Verification items for the finished model (mm, model axes). Face numbers are marked on the shaded views. A direction names the side the tool comes from. Give positions to 0.01 mm unless a question says otherwise; leave off trailing zeros. Loops run counter-clockwise (first coordinate to the right, second up) from the corner with the lowest first, then second, coordinate; pieces in that order, holes last. Notation, with made-up numbers: (-9, -20.75) -> (47, -20.75) arc R11 ccw to (47, -11.75) -> close; hole circle Ø5 at (50.25, 64). An arc over 180 degrees is marked (long way). Use one line per item in the form item = value. Start each with the question number.
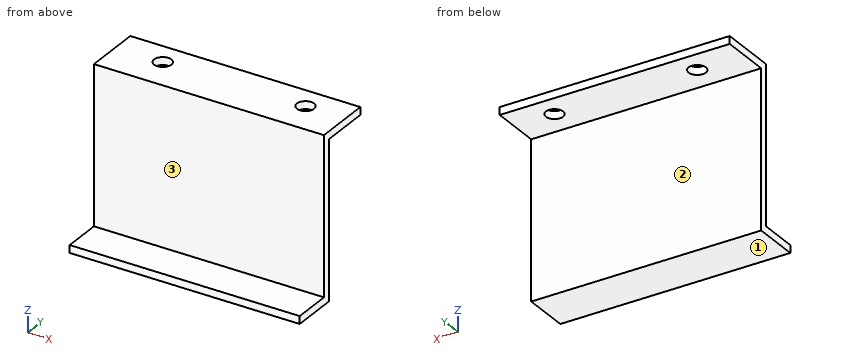
from build123d import *

# Parameters (mm, degrees)
SKETCH1_W            = 60
SKETCH1_H            = 20
BOSS_EXTRUDE1_DEPTH  = 43
SKETCH2_W            = 60
SKETCH2_H            = 8
CUT_EXTRUDE1_DEPTH   = 41
SKETCH3_W            = 60
SKETCH3_H            = 10
CUT_EXTRUDE2_DEPTH   = 41
SKETCH4_W            = 60
SKETCH4_H            = 2
BOSS_EXTRUDE2_DEPTH  = 5
M4_CLEARANCE_HOLE1_D = 4.5


with BuildPart() as part:
    # Sketch1 → Boss-Extrude1 (new body)
    with BuildSketch(Plane.XY):
        Rectangle(SKETCH1_W, SKETCH1_H)
    extrude(amount=BOSS_EXTRUDE1_DEPTH)

    # Sketch2 → Cut-Extrude1 (cut)
    with BuildSketch(Plane(origin=(0, 0, 0), x_dir=(-1, 0, 0), z_dir=(0, 0, -1))):
        with Locations((0, 6)):
            Rectangle(SKETCH2_W, SKETCH2_H)
    extrude(amount=-CUT_EXTRUDE1_DEPTH, mode=Mode.SUBTRACT)

    # Sketch3 → Cut-Extrude2 (cut)
    with BuildSketch(Plane.XY.offset(43)):
        with Locations((0, -5)):
            Rectangle(SKETCH3_W, SKETCH3_H)
    extrude(amount=-CUT_EXTRUDE2_DEPTH, mode=Mode.SUBTRACT)

    # Sketch4 → Boss-Extrude2 (add)
    with BuildSketch(Plane(origin=(0, 10, 0), x_dir=(1, 0, 0), z_dir=(0, 1, 0))):
        with Locations((0, -42)):
            Rectangle(SKETCH4_W, SKETCH4_H)
    extrude(amount=BOSS_EXTRUDE2_DEPTH)

    # M4 Clearance Hole1 (through all)
    with Locations(Plane(origin=(0, 0, 41), x_dir=(-1, 0, 0), z_dir=(0, 0, -1))):
        with Locations((-19.571160429, 8.893689212), (17.676175713, 8.893689212)):
            Hole(M4_CLEARANCE_HOLE1_D / 2)


solid = part.part
Item 1: Sectioned sample at A-A, the plane x = 23. Enter the section's corners in (y, z).
Item 2: Tool access check on the marked faces 1, 2 and 3. Record the directions out of +Z, -Z, +X, -X, +Y, -Y that give a thin tool (end or side, any length) a straight path to the whole face; none if there is none.
Item 3: Sectioned sample at B-B, the plane z = 20. Enter the section's corners in (x, y), and give its area (3 significant figures).
Item 4: Material ranges on line 1 (Z direction, x = -4, y = 7.5); line 2 (Z direction, x = 22, y = -1.25), recorded low to high.
Item 5: Gauge pin test, flat ends, axial feed: pin 1 Ø10 at (x, z) = (-21.5, 13) entering from -Y; pin 2 Ø12.5 at (x, z) = (-11.5, 17.5) entering from +Y; pin 3 Ø6 at (y, z) = (7.5, 7.5) entering from +X; pin 4 Ø4 at (x, y) = (-11.5, 11.5) entering from -Z. Record the tip position at first contact, or that the pin passes through.
Outcome:
q1.outline = (-10, 0) -> (2, 0) -> (2, 41) -> (15, 41) -> (15, 43) -> (0, 43) -> (0, 2) -> (-10, 2) -> close
q2.face_1 = -Z, +X, -X, +Y, -Y
q2.face_2 = -Z, +X, -X, +Y
q2.face_3 = +Z, +X, -X, -Y
q3.outline = (-30, 0) -> (30, 0) -> (30, 2) -> (-30, 2) -> close
q3.area = 120 mm^2
q4.line_1 = 41 to 43
q4.line_2 = 0 to 2
q5.pin_1 = 0
q5.pin_2 = 2
q5.pin_3 = through
q5.pin_4 = 41
